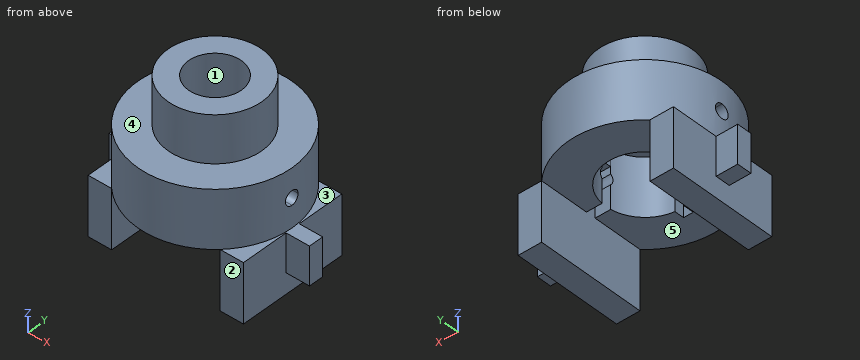
from build123d import *

# Parameters (mm, degrees)
F0_R      = 8
F0_R_2    = 4.5
F1_DEPTH  = 8
F2_R      = 13.15
F3_DEPTH  = 9.8
F4_START  = -2.8
F4_DEPTH  = 22.2
F6_DEPTH  = 10
F8_START  = -26.2
F8_DEPTH  = 4
F9_DEPTH  = 4
F10_DEPTH = 76


with BuildPart() as f1:
    # F0 (on Top) → F1 (new body)
    with BuildSketch(Plane.XY):
        Circle(F0_R)
        Circle(F0_R_2, mode=Mode.SUBTRACT)
    extrude(amount=F1_DEPTH)

    # F2 (on Top) → F3 (join)
    with BuildSketch(Plane.XY):
        Circle(F2_R)
        with BuildLine():
            ThreePointArc((-6.5986267511, 0.825), (0, 6.65), (6.5986267511, 0.825))
            Line((6.5986267511, 0.825), (6.65, 0.825))
            Line((6.65, 0.825), (9.25, 0.825))
            Line((9.25, 0.825), (9.25, -0.825))
            Line((9.25, -0.825), (6.65, -0.825))
            Line((6.65, -0.825), (6.5986267511, -0.825))
            ThreePointArc((6.5986267511, -0.825), (4.7022600949, -4.7022600949), (0.825, -6.5986267511))
            Line((0.825, -6.5986267511), (0.825, -6.65))
            Line((0.825, -6.65), (0.825, -8.25))
            Line((0.825, -8.25), (-0.825, -8.25))
            Line((-0.825, -8.25), (-0.825, -6.65))
            Line((-0.825, -6.65), (-0.825, -6.5986267511))
            ThreePointArc((-0.825, -6.5986267511), (-4.7022600949, -4.7022600949), (-6.5986267511, -0.825))
            Line((-6.5986267511, -0.825), (-6.65, -0.825))
            Line((-6.65, -0.825), (-9.25, -0.825))
            Line((-9.25, -0.825), (-9.25, 0.825))
            Line((-9.25, 0.825), (-6.65, 0.825))
            Line((-6.65, 0.825), (-6.5986267511, 0.825))
        make_face(mode=Mode.SUBTRACT)
        Polygon((-6.65, -0.825), (-6.65, 0), (-6.65, 0.825), (-9.25, 0.825), (-9.25, -0.825), align=None)
        Polygon((6.65, 0.825), (6.65, 0), (6.65, -0.825), (9.25, -0.825), (9.25, 0.825), align=None)
        Polygon((0.825, -6.65), (0, -6.65), (-0.825, -6.65), (-0.825, -8.25), (0.825, -8.25), align=None)
        with BuildLine():
            Line((0.825, -6.65), (0.825, -6.5986267511))
            ThreePointArc((0.825, -6.5986267511), (0.413298987, -6.6371442615), (0, -6.65))
            Line((0, -6.65), (0.825, -6.65))
        make_face()
        with BuildLine():
            Line((-0.825, -6.65), (0, -6.65))
            ThreePointArc((0, -6.65), (-0.413298987, -6.6371442615), (-0.825, -6.5986267511))
            Line((-0.825, -6.5986267511), (-0.825, -6.65))
        make_face()
        with BuildLine():
            ThreePointArc((6.5986267511, 0.825), (6.6371442615, 0.413298987), (6.65, 0))
            Line((6.65, 0), (6.65, 0.825))
            Line((6.65, 0.825), (6.5986267511, 0.825))
        make_face()
        with BuildLine():
            Line((6.65, -0.825), (6.65, 0))
            ThreePointArc((6.65, 0), (6.6371442615, -0.413298987), (6.5986267511, -0.825))
            Line((6.5986267511, -0.825), (6.65, -0.825))
        make_face()
        with BuildLine():
            ThreePointArc((-6.5986267511, -0.825), (-6.6371442615, -0.413298987), (-6.65, 0))
            Line((-6.65, 0), (-6.65, -0.825))
            Line((-6.65, -0.825), (-6.5986267511, -0.825))
        make_face()
        with BuildLine():
            ThreePointArc((-6.65, 0), (-6.6371442615, 0.413298987), (-6.5986267511, 0.825))
            Line((-6.5986267511, 0.825), (-6.65, 0.825))
            Line((-6.65, 0.825), (-6.65, 0))
        make_face()
    extrude(amount=-F3_DEPTH)

    # F2 (on Top) → F4 (cut)
    with BuildSketch(Plane.XY.offset(F4_START)):
        Polygon((6.65, 0.825), (6.65, 0), (6.65, -0.825), (9.25, -0.825), (9.25, 0.825), align=None)
        Polygon((0.825, -6.65), (0, -6.65), (-0.825, -6.65), (-0.825, -8.25), (0.825, -8.25), align=None)
        Polygon((-6.65, -0.825), (-6.65, 0), (-6.65, 0.825), (-9.25, 0.825), (-9.25, -0.825), align=None)
        with BuildLine():
            Line((6.65, -0.825), (6.65, 0))
            ThreePointArc((6.65, 0), (6.6371442615, -0.413298987), (6.5986267511, -0.825))
            Line((6.5986267511, -0.825), (6.65, -0.825))
        make_face()
        with BuildLine():
            ThreePointArc((6.5986267511, 0.825), (6.6371442615, 0.413298987), (6.65, 0))
            Line((6.65, 0), (6.65, 0.825))
            Line((6.65, 0.825), (6.5986267511, 0.825))
        make_face()
        with BuildLine():
            Line((-0.825, -6.65), (0, -6.65))
            ThreePointArc((0, -6.65), (-0.413298987, -6.6371442615), (-0.825, -6.5986267511))
            Line((-0.825, -6.5986267511), (-0.825, -6.65))
        make_face()
        with BuildLine():
            Line((0.825, -6.65), (0.825, -6.5986267511))
            ThreePointArc((0.825, -6.5986267511), (0.413298987, -6.6371442615), (0, -6.65))
            Line((0, -6.65), (0.825, -6.65))
        make_face()
        with BuildLine():
            ThreePointArc((-6.65, 0), (-6.6371442615, 0.413298987), (-6.5986267511, 0.825))
            Line((-6.5986267511, 0.825), (-6.65, 0.825))
            Line((-6.65, 0.825), (-6.65, 0))
        make_face()
        with BuildLine():
            ThreePointArc((-6.5986267511, -0.825), (-6.6371442615, -0.413298987), (-6.65, 0))
            Line((-6.65, 0), (-6.65, -0.825))
            Line((-6.65, -0.825), (-6.5986267511, -0.825))
        make_face()
    extrude(amount=-F4_DEPTH, mode=Mode.SUBTRACT)

    # F5 (on face) → F6 (join)
    with BuildSketch(Plane(origin=(0, 0, -9.8), x_dir=(1, 0, 0), z_dir=(0, 0, -1))):
        with BuildLine():
            ThreePointArc((13.15, 0), (12.135897165, -5.0638424146), (9.25, -9.3466571564))
            Line((9.25, -9.3466571564), (13.25, -9.3466571564))
            Line((13.25, -9.3466571564), (13.25, 9.3466571564))
            Line((13.25, 9.3466571564), (9.25, 9.3466571564))
            ThreePointArc((9.25, 9.3466571564), (12.135897165, 5.0638424146), (13.15, 0))
        make_face()
        with BuildLine():
            Line((9.25, -0.825), (9.25, -9.3466571564))
            ThreePointArc((9.25, -9.3466571564), (12.135897165, -5.0638424146), (13.15, 0))
            ThreePointArc((13.15, 0), (12.135897165, 5.0638424146), (9.25, 9.3466571564))
            Line((9.25, 9.3466571564), (9.25, 0.825))
            Line((9.25, 0.825), (9.25, -0.825))
        make_face()
        with BuildLine():
            ThreePointArc((-9.25, 9.3466571564), (-13.15, 0), (-9.25, -9.3466571564))
            Line((-9.25, -9.3466571564), (-9.25, -0.825))
            Line((-9.25, -0.825), (-9.25, 0.825))
            Line((-9.25, 0.825), (-9.25, 9.3466571564))
        make_face()
        with BuildLine():
            Line((-13.25, -9.3466571564), (-9.25, -9.3466571564))
            ThreePointArc((-9.25, -9.3466571564), (-13.15, 0), (-9.25, 9.3466571564))
            Line((-9.25, 9.3466571564), (-13.25, 9.3466571564))
            Line((-13.25, 9.3466571564), (-13.25, -9.3466571564))
        make_face()
    extrude(amount=F6_DEPTH)

    # F7 (on face) → F8 (join)
    with BuildSketch(Plane.YZ.offset(13.25).offset(F8_START)):
        Polygon((0, -9.8), (-1.25, -9.8), (-1.25, -16.3), (1.25, -16.3), (1.25, -9.8), align=None)
    extrude(amount=-F8_DEPTH)

    # F7 (on face) → F9 (join)
    with BuildSketch(Plane.YZ.offset(13.25)):
        Polygon((0, -9.8), (-1.25, -9.8), (-1.25, -16.3), (1.25, -16.3), (1.25, -9.8), align=None)
    extrude(amount=F9_DEPTH)

    # F7 (on face) → F10 (cut)
    with BuildSketch(Plane.YZ.offset(13.25)):
        with BuildLine():
            ThreePointArc((0, -3.7), (-1.2, -4.9), (0, -6.1))
            Line((0, -6.1), (0, -3.7))
        make_face()
        with BuildLine():
            Line((0, -3.7), (0, -6.1))
            ThreePointArc((0, -6.1), (0.8485281374, -5.7485281374), (1.2, -4.9))
            ThreePointArc((1.2, -4.9), (0.8485281374, -4.0514718626), (0, -3.7))
        make_face()
    extrude(amount=-F10_DEPTH, mode=Mode.SUBTRACT)


solid = f1.part
Read the model definition and answer for the solid it produces. Units are mm, in the model's axes. Face numbers are marked on the shaded views. A direction names the side the tool comes from. Coordinates: 2 decimals unless noted, no trailing zeros. Write each loop counter-clockwise with the first axis right and the second up, starting at its lowest first coordinate (ties: lowest second). Pieces come first, ordered by that corner, then holes. Notation, with made-up numbers: (-29.75, 76.5) -> (-19.75, 76.5) arc R13 ccw to (-19.75, 85.5) -> close; hole circle Ø5 at (21.5, -17.5). An arc over 180 degrees is marked (long way). Return JSON: item names as keys, results as strings.
(1) Consider line 1 along X through (y, z) = (0, -11.75); line 2 along X through (y, z) = (-7.5, -10.25); line 3 along Y through (x, z) = (0, 5.25). Determine where each line is inside the solid, lowest interval first. Write a range as from..to.
Answers below:
{"line 1": "-16.95..-9.25, 9.25..17.25", "line 2": "-13.25..-9.25, 9.25..13.25", "line 3": "-8..-4.5, 4.5..8"}
(2) Which of the six approach directions +Z, -Z, +X, -X, +Y, -Y give full straight-line access (tool end or side, diameter ignored) to the marked faces 1, 2, 3, 4 and 5?
Answers below:
{"face 1": "+Z, -Z", "face 2": "+Z, -Z, +X, -X, -Y", "face 3": "+Z, +X", "face 4": "+Z", "face 5": "-Z, +Y, -Y"}
(3) The part is cut by section D-D on x = -14. Give the vertices of the cut face in (y, z), then the cut area to 4 significant figures.
Answers below:
{"outline": "(-1.25, -16.3) -> (1.25, -16.3) -> (1.25, -9.8) -> (-1.25, -9.8) -> close", "area": "16.25 mm^2"}
(4) The part is cut by section A-A on z = -15.25. Give the vertices of the cut face in (x, y), then the cut area to 3 significant figures.
Answers below:
{"outline": "(-16.95, -1.25) -> (-13.25, -1.25) -> (-13.25, -9.35) -> (-9.25, -9.35) -> (-9.25, 9.35) -> (-13.25, 9.35) -> (-13.25, 1.25) -> (-16.95, 1.25) -> close; (9.25, -9.35) -> (13.25, -9.35) -> (13.25, -1.25) -> (17.25, -1.25) -> (17.25, 1.25) -> (13.25, 1.25) -> (13.25, 9.35) -> (9.25, 9.35) -> close", "area": "169 mm^2"}
(5) The part is cut by section B-B on z = -8. Give the vertices of the cut face in (x, y) (3 decimals).
Answers below:
{"outline": "circle Ø26.3 at (0, 0); hole (-9.25, -0.825) -> (-6.599, -0.825) arc R6.65 ccw to (-0.825, -6.599) -> (-0.825, -8.25) -> (0.825, -8.25) -> (0.825, -6.599) arc R6.65 ccw to (6.599, -0.825) -> (9.25, -0.825) -> (9.25, 0.825) -> (6.599, 0.825) arc R6.65 ccw to (-6.599, 0.825) -> (-9.25, 0.825) -> close"}
(6) Each of these flat-tipped pins is pushed along its axis until it touches: P1, Ø4, axis at x = 12, y = 4, coming from the +Z side; P2, Ø5, axis at x = 9, y = 7.5, coming from the -Z side; P3, Ø2, axis at y = 10, z = 2, coming from the -X side; P4, Ø1.4, axis at x = 7.5, z = -3.5, coming from the +Y side. Where does it stop, or does it pass through?
Answers below:
{"P1": "z = 0", "P2": "z = -19.8", "P3": "through", "P4": "y = 11.26"}
(7) The part is cut by section C-C on y = 2.75. Give the vertices of the cut face in (x, z).
Answers below:
{"outline": "(-13.25, -19.8) -> (-9.25, -19.8) -> (-9.25, -9.8) -> (-6.05, -9.8) -> (-6.05, 0) -> (-3.56, 0) -> (-3.56, 8) -> (-7.51, 8) -> (-7.51, 0) -> (-12.86, 0) -> (-12.86, -9.8) -> (-13.25, -9.8) -> close; (3.56, 0) -> (6.05, 0) -> (6.05, -9.8) -> (9.25, -9.8) -> (9.25, -19.8) -> (13.25, -19.8) -> (13.25, -9.8) -> (12.86, -9.8) -> (12.86, 0) -> (7.51, 0) -> (7.51, 8) -> (3.56, 8) -> close"}
